from build123d import *

# Parameters (mm, degrees)
BOX004_W          = 40
BOX004_H          = 40
BOX004_DEPTH      = 10
CYLINDER009_R     = 1.6
CYLINDER009_DEPTH = 20
CYLINDER008_R     = 1.6
CYLINDER008_DEPTH = 20
CYLINDER007_R     = 1.6
CYLINDER007_DEPTH = 20
CYLINDER006_R     = 1.6
CYLINDER006_DEPTH = 10
CYLINDER005_R     = 1.6
CYLINDER005_DEPTH = 10
CYLINDER004_R     = 1.6
CYLINDER004_DEPTH = 10
BOX003_W          = 10
BOX003_H          = 40
BOX003_DEPTH      = 14
BOX002_W          = 11.5
BOX002_H          = 40
BOX002_DEPTH      = 4
BOX001_W          = 17.5
BOX001_H          = 40
BOX001_DEPTH      = 2.75
CYLINDER003_R     = 1.5
CYLINDER003_DEPTH = 10
CYLINDER002_R     = 1.5
CYLINDER002_DEPTH = 10
CYLINDER001_R     = 1.5
CYLINDER001_DEPTH = 10
CYLINDER_R        = 1.5
CYLINDER_DEPTH    = 10
BOX_W             = 90
BOX_H             = 90
BOX_DEPTH         = 2.5


with BuildPart() as cube004:
    # Box004 → Box004 (new body)
    with BuildSketch(Plane(origin=(53, 50, -5), x_dir=(1, 0, 0), z_dir=(0, 0, 1))):
        with Locations((20, 20)):
            Rectangle(BOX004_W, BOX004_H)
    extrude(amount=BOX004_DEPTH)


with BuildPart() as cylinder009:
    # Cylinder009 → Cylinder009 (new body)
    with BuildSketch(Plane(origin=(50, 70, -5), x_dir=(1, 0, 0), z_dir=(0, 0, 1))):
        Circle(CYLINDER009_R)
    extrude(amount=CYLINDER009_DEPTH)


with BuildPart() as cylinder008:
    # Cylinder008 → Cylinder008 (new body)
    with BuildSketch(Plane(origin=(39, 70, -5), x_dir=(1, 0, 0), z_dir=(0, 0, 1))):
        Circle(CYLINDER008_R)
    extrude(amount=CYLINDER008_DEPTH)


with BuildPart() as cylinder007:
    # Cylinder007 → Cylinder007 (new body)
    with BuildSketch(Plane(origin=(39, 65, -5), x_dir=(1, 0, 0), z_dir=(0, 0, 1))):
        Circle(CYLINDER007_R)
    extrude(amount=CYLINDER007_DEPTH)


with BuildPart() as cylinder006:
    # Cylinder006 → Cylinder006 (new body)
    with BuildSketch(Plane(origin=(27, 65, -5), x_dir=(1, 0, 0), z_dir=(0, 0, 1))):
        Circle(CYLINDER006_R)
    extrude(amount=CYLINDER006_DEPTH)


with BuildPart() as cylinder005:
    # Cylinder005 → Cylinder005 (new body)
    with BuildSketch(Plane(origin=(27, 70, -5), x_dir=(1, 0, 0), z_dir=(0, 0, 1))):
        Circle(CYLINDER005_R)
    extrude(amount=CYLINDER005_DEPTH)


with BuildPart() as cylinder004:
    # Cylinder004 → Cylinder004 (new body)
    with BuildSketch(Plane(origin=(9, 70, -5), x_dir=(1, 0, 0), z_dir=(0, 0, 1))):
        Circle(CYLINDER004_R)
    extrude(amount=CYLINDER004_DEPTH)


with BuildPart() as cube003:
    # Box003 → Box003 (new body)
    with BuildSketch(Plane(origin=(39, 50, 0), x_dir=(1, 0, 0), z_dir=(0, 0, 1))):
        with Locations((5, 20)):
            Rectangle(BOX003_W, BOX003_H)
    extrude(amount=BOX003_DEPTH)


with BuildPart() as cube002:
    # Box002 → Box002 (new body)
    with BuildSketch(Plane(origin=(27.5, 50, 0), x_dir=(1, 0, 0), z_dir=(0, 0, 1))):
        with Locations((5.75, 20)):
            Rectangle(BOX002_W, BOX002_H)
    extrude(amount=BOX002_DEPTH)


with BuildPart() as cube001:
    # Box001 → Box001 (new body)
    with BuildSketch(Plane(origin=(10, 50, 0), x_dir=(1, 0, 0), z_dir=(0, 0, 1))):
        with Locations((8.75, 20)):
            Rectangle(BOX001_W, BOX001_H)
    extrude(amount=BOX001_DEPTH)


with BuildPart() as cylinder003:
    # Cylinder003 → Cylinder003 (new body)
    with BuildSketch(Plane(origin=(83, 45, -5), x_dir=(1, 0, 0), z_dir=(0, 0, 1))):
        Circle(CYLINDER003_R)
    extrude(amount=CYLINDER003_DEPTH)


with BuildPart() as cylinder002:
    # Cylinder002 → Cylinder002 (new body)
    with BuildSketch(Plane(origin=(83, 5, -5), x_dir=(1, 0, 0), z_dir=(0, 0, 1))):
        Circle(CYLINDER002_R)
    extrude(amount=CYLINDER002_DEPTH)


with BuildPart() as cylinder001:
    # Cylinder001 → Cylinder001 (new body)
    with BuildSketch(Plane(origin=(7, 45, -5), x_dir=(1, 0, 0), z_dir=(0, 0, 1))):
        Circle(CYLINDER001_R)
    extrude(amount=CYLINDER001_DEPTH)


with BuildPart() as cylinder:
    # Cylinder → Cylinder (new body)
    with BuildSketch(Plane(origin=(7, 5, -5), x_dir=(1, 0, 0), z_dir=(0, 0, 1))):
        Circle(CYLINDER_R)
    extrude(amount=CYLINDER_DEPTH)


with BuildPart() as cut010:
    # Box → Box (new body)
    with BuildSketch(Plane.XY.offset(-2.5)):
        with Locations((45, 45)):
            Rectangle(BOX_W, BOX_H)
    extrude(amount=BOX_DEPTH)

    # Cut: cut Cylinder
    add(cylinder.part, mode=Mode.SUBTRACT)

    # Cut001: cut Cylinder001
    add(cylinder001.part, mode=Mode.SUBTRACT)

    # Cut002: cut Cylinder002
    add(cylinder002.part, mode=Mode.SUBTRACT)

    # Cut003: cut Cylinder003
    add(cylinder003.part, mode=Mode.SUBTRACT)

    # Fusion: union Cube001
    add(cube001.part)

    # Fusion001: union Cube002
    add(cube002.part)

    # Fusion002: union Cube003
    add(cube003.part)

    # Cut004: cut Cylinder004
    add(cylinder004.part, mode=Mode.SUBTRACT)

    # Cut005: cut Cylinder005
    add(cylinder005.part, mode=Mode.SUBTRACT)

    # Cut006: cut Cylinder006
    add(cylinder006.part, mode=Mode.SUBTRACT)

    # Cut007: cut Cylinder007
    add(cylinder007.part, mode=Mode.SUBTRACT)

    # Cut008: cut Cylinder008
    add(cylinder008.part, mode=Mode.SUBTRACT)

    # Cut009: cut Cylinder009
    add(cylinder009.part, mode=Mode.SUBTRACT)

    # Cut010: cut Cube004
    add(cube004.part, mode=Mode.SUBTRACT)


solid = cut010.part
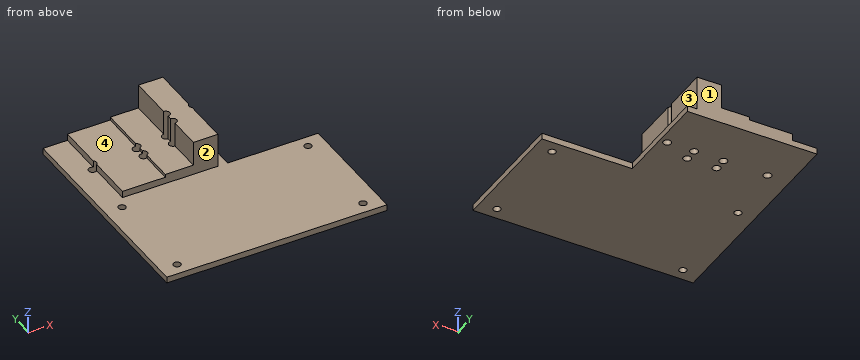
The listing builds one solid part. Answer for the finished solid, in the listing's coordinates (mm). Face numbers are marked on the shaded views. A direction names the side the tool comes from. Give positions to 0.01 mm unless a question says otherwise; leave off trailing zeros. Write each loop counter-clockwise with the first axis right and the second up, starting at its lowest first coordinate (ties: lowest second). Pieces come first, ordered by that corner, then holes. Notation, with made-up numbers: (-4.5, 54) - (2.5, 54) arc R21 cw to (2.5, 82) - close; hole circle Ø4 at (63.5, 62). An arc over 180 degrees is marked (long way). One line per question, with ' | ' between items. Start each with the question number.
1. For the marked faces 1, 2, 3 and 4, determine the directions among +Z, -Z, +X, -X, +Y, -Y from which every point of the face is accessible in a straight line to the end or side of a thin tool.
2. Section C-C, the plane z = 10 is taken. Determine the outline of the cut face in (x, y).
3. Straight lines are drawn through the part: line 1 (Y direction, x = 7, z = -1.1); line 2 (Y direction, x = 27, z = 0.75); line 3 (X direction, y = 5, z = -1.8). For each, find the intervals that lie inside material, in ascending order.
4. Given P1, Ø1.5, axis at y = 59, z = 9, coming from the +X side; P2, Ø0.8, axis at y = 68, z = -1, coming from the +X side; P3, Ø1, axis at x = 29.5, z = 2, coming from the -Y side, each flat-ended and moving along its own axis, determine where each tip first touches the part or whether it passes through.
5. Section B-B, the plane y = 5 is taken. Determine the outline of the cut face in (x, z), then the cut area to 3 significant figures.
6. Section A-A, the plane y = 70 is taken. Determine the outline of the cut face in (x, z), then the cut area to 3 significant figures.
7. Section D-D, the plane x = 12 is taken. Determine the outline of the cut face in (y, z).
Result:
1) face 1: +Z, -Z, +X, -X, +Y | face 2: +Z, +X, -X, -Y | face 3: +Z, +X, +Y, -Y | face 4: +Z, -X, +Y, -Y
2) outline: (39, 50) - (49, 50) - (49, 68.75) arc R1.6 cw to (49, 71.25) - (49, 90) - (39, 90) - (39, 71.6) arc R1.6 cw to (39, 68.4) - (39, 66.6) arc R1.6 cw to (39, 63.4) - close
3) line 1: y = 0 to 3.5, 6.5 to 43.5, 46.5 to 90 | line 2: y = 50 to 63.4, 66.6 to 68.4, 71.6 to 90 | line 3: x = 0 to 5.5, 8.5 to 81.5, 84.5 to 90
4) P1: stops at x = 49 | P2: stops at x = 53 | P3: stops at y = 50
5) outline: (0, -2.5) - (5.5, -2.5) - (5.5, 0) - (0, 0) - close; (8.5, -2.5) - (81.5, -2.5) - (81.5, 0) - (8.5, 0) - close; (84.5, -2.5) - (90, -2.5) - (90, 0) - (84.5, 0) - close | area: 210 mm2
6) outline: (0, -2.5) - (7.4, -2.5) - (7.4, 0) - (0, 0) - close; (10.6, -2.5) - (25.4, -2.5) - (25.4, 2.75) - (10.6, 2.75) - close; (28.6, -2.5) - (37.4, -2.5) - (37.4, 4) - (28.6, 4) - close; (40.6, -2.5) - (48.4, -2.5) - (48.4, 14) - (40.6, 14) - close; (51.6, -2.5) - (53, -2.5) - (53, 0) - (51.6, 0) - close | area: 286 mm2
7) outline: (0, -2.5) - (90, -2.5) - (90, 2.75) - (50, 2.75) - (50, 0) - (0, 0) - close
